The listing builds one solid part. Answer for the finished solid, in the listing's coordinates (mm). A direction names the side the tool comes from. Round coordinates to 2 decimals unless told otherwise and drop trailing zeros. Write each loop counter-clockwise with the first axis right and the second up, starting at its lowest first coordinate (ties: lowest second). Pieces come first, ordered by that corner, then holes.
from build123d import *

# Parameters (mm, degrees)
SKETCH1_R           = 1.2
BOSS_EXTRUDE1_DEPTH = 4
FILLET1_R           = 7
FILLET2_START       = -1
FILLET2_DEPTH       = 6


with BuildPart() as part:
    # Sketch1 → Boss-Extrude1 (new body)
    with BuildSketch(Plane.XY):
        with BuildLine():
            Line((8, 37.42), (8, 32.42))
            Line((8, 32.42), (0, 32.42))
            Line((0, 32.42), (0, 27.42))
            Line((0, 27.42), (4, 27.42))
            Line((4, 27.42), (4, 19.42))
            Line((4, 19.42), (0, 19.42))
            Line((0, 19.42), (0, 0))
            Line((0, 0), (13.75, 0))
            ThreePointArc((13.75, 0), (32.824339015, -13.98588401), (25.221528727, -36.383040886))
            Line((25.221528727, -36.383040886), (30.957293091, -44.574561329))
            ThreePointArc((30.957293091, -44.574561329), (43.681938755, -17.980336071), (27.5, 6.66341126))
            Line((27.5, 6.66341126), (27.5, 19.42))
            Line((27.5, 19.42), (23.5, 19.42))
            Line((23.5, 19.42), (23.5, 27.42))
            Line((23.5, 27.42), (27.5, 27.42))
            Line((27.5, 27.42), (27.5, 32.42))
            Line((27.5, 32.42), (19.5, 32.42))
            Line((19.5, 32.42), (19.5, 37.42))
            Line((19.5, 37.42), (8, 37.42))
        make_face()
        with Locations((3, 13)):
            Circle(SKETCH1_R, mode=Mode.SUBTRACT)
        with BuildLine():
            ThreePointArc((16.590873036, 15.687904348), (13.75, 12.61), (10.909126964, 15.687904348))
            ThreePointArc((10.909126964, 15.687904348), (13.75, 27.42), (16.590873036, 15.687904348))
        make_face(mode=Mode.SUBTRACT)
        with Locations((13.75, 34.42)):
            Circle(SKETCH1_R, mode=Mode.SUBTRACT)
        with Locations((23.5, 13)):
            Circle(SKETCH1_R, mode=Mode.SUBTRACT)
    extrude(amount=BOSS_EXTRUDE1_DEPTH)

    # Fillet1
    fillet1_edges = [part.edges().sort_by_distance(p)[0] for p in [
        (27.5, 6.66341126, 2),
        (0, 0, 2),
    ]]
    fillet(fillet1_edges, radius=FILLET1_R)

    # Fillet2: read off the stored shape, not the designer's step
    # Fillet2 outline → Fillet2 (cut)
    with BuildSketch(Plane.XY.offset(FILLET2_START)):
        with BuildLine():
            ThreePointArc((30.957293091, -44.574561329), (33.340121642, -42.720632343), (35.524547437, -40.636595745))
            add(Edge.make_bspline(
                [(35.524547437, -40.636595745), (34.55329691, -41.661403369), (33.063664011, -42.522816758), (31.099164619, -42.770231906), (29.107575632, -41.932891027), (27.799695976, -40.065045303)],
                knots=[0, 0, 0, 0, 0, 0, 0.550510257, 0.550510257, 0.550510257, 0.550510257, 0.550510257, 0.550510257], degree=5, weights=[1, 0.779795897, 0.620204103, 0.521224617, 0.48285744, 0.505102572]))
            Line((27.799695976, -40.065045303), (30.957293091, -44.574561329))
        make_face()
        with BuildLine():
            Line((25.221528727, -36.383040886), (27.799695976, -40.065045303))
            add(Edge.make_bspline(
                [(27.799695976, -40.065045303), (26.814281677, -38.657727837), (26.550577461, -37.082538129), (26.869269697, -35.66327749), (27.512411311, -34.553258967), (28.266364958, -33.757730497)],
                knots=[0.550510257, 0.550510257, 0.550510257, 0.550510257, 0.550510257, 0.550510257, 1, 1, 1, 1, 1, 1], degree=5, weights=[0.505102572, 0.523265646, 0.581836926, 0.680816412, 0.820204103, 1]))
            ThreePointArc((28.266364958, -33.757730497), (26.810081095, -35.147088229), (25.221528727, -36.383040886))
        make_face()
    extrude(amount=FILLET2_DEPTH, mode=Mode.SUBTRACT)


solid = part.part
1. Given pin 1 (2 mm diameter, centred on y = 30.5, z = 2, fed in from +X); pin 2 (1.2 mm diameter, centred on x = 5, z = 2.5, fed in from +Y); pin 3 (1 mm diameter, centred on x = 33, z = 2, fed in from -Y), each flat-ended and moving along its own axis, determine where each tip first touches the part or whether it passes through.
Geometry says:
pin 1: stops at x = 27.5
pin 2: stops at y = 32.42
pin 3: stops at y = -42.16
2. Section B-B on x = 3 is taken. Determine the outline of the cut face in (y, z), plus the area to 3 significant figures.
Geometry says:
outline: (1.26, 0) - (11.8, 0) - (11.8, 4) - (1.26, 4) - close; (14.2, 0) - (19.42, 0) - (19.42, 4) - (14.2, 4) - close; (27.42, 0) - (32.42, 0) - (32.42, 4) - (27.42, 4) - close
area: 83.1 mm2
3. Section D-D on z = 1.65 is taken. Give the number of separate pieces and of enclosed holes in the cut face, plus the area to 3 significant figures.
Geometry says:
separate pieces: 1
enclosed holes: 4
area: 1,230 mm2
4. For a pull along Y with two mould halves and no side action, classify faces 5 (the face through (2.74, 11.83, 1.97)), 6 (the face through (24, 32.42, 2)), 7 (the face through (27.5, 30, 2)) as released by +Y, released by -Y, zero draft, split by the parting line, or undercut.
Geometry says:
face 5: undercut
face 6: released by +Y
face 7: zero draft
5. Section A-A on y = 34.42 is taken. Determine the outline of the cut face in (x, z).
Geometry says:
outline: (8, 0) - (12.55, 0) - (12.55, 4) - (8, 4) - close; (14.95, 0) - (19.5, 0) - (19.5, 4) - (14.95, 4) - close
6. A tool of negligible diameter and unlimited length cuts with its end or side. For faces 1 (the face through (10, 0, 2)), 2 (the face through (19.5, 35, 2)), 3 (the face through (23.5, 23, 2)), 4 (the face through (2, 27.42, 2)), from which of +Z, -Z, +X, -X, +Y, -Y can it reach the whole face along a straight path? Write none if from no direction.
Geometry says:
face 1: +Z, -Z, -X, -Y
face 2: +Z, -Z, +X, +Y
face 3: +Z, -Z, +X
face 4: +Z, -Z, -X
7. Straight lines are drawn through the part: line 1 along Y through (x, z) = (13.75, 1.1); line 2 along X through (y, z) = (21.21, 2.3); line 3 along X through (y, z) = (14, 1.95). For each, find the intervals that lie inside material, in ascending order.
Geometry says:
line 1: y = 0 to 12.61, 27.42 to 33.22, 35.62 to 37.42
line 2: x = 4 to 7.54, 19.96 to 23.5
line 3: x = 0 to 2.34, 3.66 to 11.3, 16.2 to 22.84, 24.16 to 27.5
8. Section C-C on x = 25.5 is taken. Determine the outline of the cut face in (y, z), plus the area to 3 significant figures.
Geometry says:
outline: (-3.82, 0) - (19.42, 0) - (19.42, 4) - (-3.82, 4) - close; (27.42, 0) - (32.42, 0) - (32.42, 4) - (27.42, 4) - close
area: 113 mm2
